Build history of the part. All positions in model axes, mm. Face numbers are marked on the shaded views. Give positions to 0.01 mm unless a question says otherwise; leave off trailing zeros. Write each loop counter-clockwise with the first axis right and the second up, starting at its lowest first coordinate (ties: lowest second). Pieces come first, ordered by that corner, then holes. Notation, with made-up numbers: (18, 84.5) -> (64, 84.5) arc R25 ccw to (64, 101.5) -> close; hole circle Ø4 at (78, 49). An arc over 180 degrees is marked (long way). One line per question, with ' | ' between items. Start each with the question number.
(1) Drill centre lines: probe 1 along Y at (x, z) = (25, 1.7); probe 2 along X at (y, z) = (-75, 1.3); probe 3 along Y at (x, z) = (14, 1.5). Where is each one in solid material? Low to high. Write a range as from..to.
(2) Pull direction Y, two halves, no side cores. Call the marked faces 1 and 2: released by +Y, released by -Y, zero draft, split by the parting line, or undercut.
(3) Band-saw the part on D-D, the plane x = 65. Give the cut face in (y, z).
(4) Band-saw the part on A-A, the plane x = 40.5. Count the separate pieces of the cut face and the enclosed holes in it, and give its area (3 significant figures).
(5) Band-saw the part on B-B, the plane y = -146. Give the cut face in (x, z), and give its area (3 significant figures).
(6) Pin check, flat tips, straight feed: P1, Ø4.5, axis at x = 5, y = -75, coming from the -Z side; P2, Ø4.5, axis at x = 76, y = -75, coming from the +Z side; P3, Ø1.9, axis at x = 25, y = -32.5, coming from the -Z side; P4, Ø7, axis at x = 79, y = -90, coming from the -Z side. Stop position of each tip, or through.
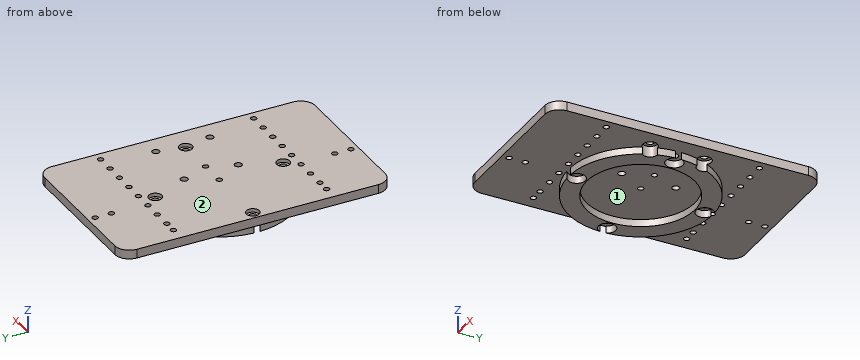
from build123d import *

# Parameters (mm, degrees)
SKETCH_1_W          = 90
SKETCH_1_H          = 150
SKETCH_1_R          = 2
SKETCH_1_R_2        = 2.15
SKETCH_1_R_3        = 1.6
EXTRUDE_1_DEPTH     = 5
FILLET_1_R          = 8
SKETCH_2_R          = 3.6
CUT_EXTRUDE_1_DEPTH = 2
SKETCH_4_R          = 30
EXTRUDE_2_DEPTH     = 4
SKETCH_5_R          = 4
CUT_EXTRUDE_2_DEPTH = 6


with BuildPart() as part:
    # 草图1 → 凸台-拉伸1 (new body)
    with BuildSketch(Plane.XY):
        with Locations((45, -75)):
            Rectangle(SKETCH_1_W, SKETCH_1_H)
        with Locations((79, -60)):
            Circle(SKETCH_1_R, mode=Mode.SUBTRACT)
        with Locations((79, -90)):
            Circle(SKETCH_1_R, mode=Mode.SUBTRACT)
        with Locations((49, -60)):
            Circle(SKETCH_1_R, mode=Mode.SUBTRACT)
        with Locations((49, -90)):
            Circle(SKETCH_1_R, mode=Mode.SUBTRACT)
        with Locations((40.5, -39.5)):
            Circle(SKETCH_1_R_2, mode=Mode.SUBTRACT)
        with Locations((40.5, -110.5)):
            Circle(SKETCH_1_R_2, mode=Mode.SUBTRACT)
        with Locations((76, -75)):
            Circle(SKETCH_1_R_2, mode=Mode.SUBTRACT)
        with Locations((5, -75)):
            Circle(SKETCH_1_R_2, mode=Mode.SUBTRACT)
        with Locations((85, -117.5)):
            Circle(SKETCH_1_R_3, mode=Mode.SUBTRACT)
        with Locations((75, -117.5)):
            Circle(SKETCH_1_R_3, mode=Mode.SUBTRACT)
        with Locations((65, -117.5)):
            Circle(SKETCH_1_R_3, mode=Mode.SUBTRACT)
        with Locations((55, -117.5)):
            Circle(SKETCH_1_R_3, mode=Mode.SUBTRACT)
        with Locations((45, -117.5)):
            Circle(SKETCH_1_R_3, mode=Mode.SUBTRACT)
        with Locations((85, -32.5)):
            Circle(SKETCH_1_R_3, mode=Mode.SUBTRACT)
        with Locations((75, -32.5)):
            Circle(SKETCH_1_R_3, mode=Mode.SUBTRACT)
        with Locations((65, -32.5)):
            Circle(SKETCH_1_R_3, mode=Mode.SUBTRACT)
        with Locations((55, -32.5)):
            Circle(SKETCH_1_R_3, mode=Mode.SUBTRACT)
        with Locations((45, -32.5)):
            Circle(SKETCH_1_R_3, mode=Mode.SUBTRACT)
        with Locations((35, -117.5)):
            Circle(SKETCH_1_R_3, mode=Mode.SUBTRACT)
        with Locations((25, -117.5)):
            Circle(SKETCH_1_R_3, mode=Mode.SUBTRACT)
        with Locations((15, -117.5)):
            Circle(SKETCH_1_R_3, mode=Mode.SUBTRACT)
        with Locations((35, -32.5)):
            Circle(SKETCH_1_R_3, mode=Mode.SUBTRACT)
        with Locations((25, -32.5)):
            Circle(SKETCH_1_R_3, mode=Mode.SUBTRACT)
        with Locations((15, -32.5)):
            Circle(SKETCH_1_R_3, mode=Mode.SUBTRACT)
        with Locations((8, -117.5)):
            Circle(SKETCH_1_R_3, mode=Mode.SUBTRACT)
        with Locations((8, -32.5)):
            Circle(SKETCH_1_R_3, mode=Mode.SUBTRACT)
        with Locations((36.5, -4)):
            Circle(SKETCH_1_R_3, mode=Mode.SUBTRACT)
        with Locations((36.5, -13)):
            Circle(SKETCH_1_R_3, mode=Mode.SUBTRACT)
        with Locations((36.5, -137)):
            Circle(SKETCH_1_R_3, mode=Mode.SUBTRACT)
        with Locations((36.5, -146)):
            Circle(SKETCH_1_R_3, mode=Mode.SUBTRACT)
        with Locations((55, -75)):
            Circle(SKETCH_1_R_3, mode=Mode.SUBTRACT)
        with Locations((40.5, -75)):
            Circle(SKETCH_1_R_3, mode=Mode.SUBTRACT)
    extrude(amount=EXTRUDE_1_DEPTH)

    # 圆角1
    fillet_1_edges = [part.edges().sort_by_distance(p)[0] for p in [
        (0, 0, 2.5),
        (90, 0, 2.5),
        (90, -150, 2.5),
        (0, -150, 2.5),
    ]]
    fillet(fillet_1_edges, radius=FILLET_1_R)

    # 草图2 → 切除-拉伸1 (cut)
    with BuildSketch(Plane.XY.offset(5)):
        with Locations((40.5, -39.5)):
            Circle(SKETCH_2_R)
        with Locations((76, -75)):
            Circle(SKETCH_2_R)
        with Locations((5, -75)):
            Circle(SKETCH_2_R)
        with Locations((40.5, -110.5)):
            Circle(SKETCH_2_R)
    extrude(amount=-CUT_EXTRUDE_1_DEPTH, mode=Mode.SUBTRACT)

    # 草图4 → 凸台-拉伸2 (add)
    with BuildSketch(Plane(origin=(0, 0, 0), x_dir=(-1, 0, 0), z_dir=(0, 0, -1))):
        with BuildLine():
            ThreePointArc((-42.199612772, -35.036124857), (-68.784271247, -46.715728753), (-80.463875143, -73.300387228))
            ThreePointArc((-80.463875143, -73.300387228), (-71.223509147, -75), (-80.463875143, -76.699612772))
            ThreePointArc((-80.463875143, -76.699612772), (-68.784271247, -103.284271247), (-42.199612772, -114.963875143))
            ThreePointArc((-42.199612772, -114.963875143), (-40.5, -105.723509147), (-38.800387228, -114.963875143))
            ThreePointArc((-38.800387228, -114.963875143), (-12.215728753, -103.284271247), (-0.536124857, -76.699612772))
            ThreePointArc((-0.536124857, -76.699612772), (-9.776490853, -75), (-0.536124857, -73.300387228))
            ThreePointArc((-0.536124857, -73.300387228), (-12.215728753, -46.715728753), (-38.800387228, -35.036124857))
            ThreePointArc((-38.800387228, -35.036124857), (-40.5, -44.276490853), (-42.199612772, -35.036124857))
        make_face()
        with Locations((-40.5, -75)):
            Circle(SKETCH_4_R, mode=Mode.SUBTRACT)
    extrude(amount=EXTRUDE_2_DEPTH)

    # 草图5 → 切除-拉伸2 (cut)
    with BuildSketch(Plane(origin=(0, 0, -4), x_dir=(-1, 0, 0), z_dir=(0, 0, -1))):
        with Locations((-79, -60)):
            Circle(SKETCH_5_R)
        with Locations((-79, -90)):
            Circle(SKETCH_5_R)
    extrude(amount=-CUT_EXTRUDE_2_DEPTH, mode=Mode.SUBTRACT)


solid = part.part
Results:
1) probe 1: y = -150..-119.1, -115.9..-34.1, -30.9..0 | probe 2: x = 0..2.85, 7.15..38.9, 42.1..53.4, 56.6..73.85, 78.15..90 | probe 3: y = -150..-118.75, -116.25..-33.75, -31.25..0
2) face 1: undercut | face 2: zero draft
3) outline: (-150, 0) -> (-119.1, 0) -> (-119.1, 5) -> (-150, 5) -> close; (-115.9, 0) -> (-106.62, 0) -> (-106.62, -4) -> (-92.31, -4) -> (-92.31, 0) -> (-57.69, 0) -> (-57.69, -4) -> (-43.38, -4) -> (-43.38, 0) -> (-34.1, 0) -> (-34.1, 5) -> (-115.9, 5) -> close; (-30.9, 0) -> (0, 0) -> (0, 5) -> (-30.9, 5) -> close
4) separate pieces: 4 | enclosed holes: 0 | area: 685 mm²
5) outline: (1.07, 0) -> (34.9, 0) -> (34.9, 5) -> (1.07, 5) -> close; (38.1, 0) -> (88.93, 0) -> (88.93, 5) -> (38.1, 5) -> close | area: 423 mm²
6) P1: stops at z = 0 | P2: stops at z = 3 | P3: passes through | P4: stops at z = 2
